Input: part model. Units: mm. Frame: model coordinates. A direction names the side the tool comes from. Coordinates: 2 decimals unless noted, no trailing zeros. Loops run counter-clockwise (first coordinate to the right, second up) from the corner with the lowest first, then second, coordinate; pieces in that order, holes last. Notation, with made-up numbers: M 31,29.5 L 36,29.5 A15 ccw 36,47.5 Z; hole C 20.5,-23.75 d4. An arc over 180 degrees is marked long. Use a Markdown table: item, result. Add a question column.
1. Section B-B on y = 0.95. Output: boundary loops of the cut face in (x, z), then the cut area to 3 significant figures.
2. Pin query (flat end, axial travel): pin 1 (18 mm diameter, centred on x = -1.5, z = 7, fed in from +Y); pin 2 (1 mm diameter, centred on y = 2.5, z = 16, fed in from +X). Return the tip coordinate at first contact, or that it passes through.
3. Line query: L1, parallel to X at y = 0.45, z = -15.25; L2, parallel to X at y = 0.35, z = -14.5. Output: solid intervals per line, ascending. Write a range as [from, to].
4. Section A-A on x = 15.25. Output: boundary loops of the cut face in (y, z).
5. Section C-C on z = -0.5. Output: boundary loops of the cut face in (x, y).
6. Set-up query: faces 5 (the flat face through (9, 3, 14.998)), 6 (the cylindrical face through (-16.75, 0.86, 15.18)). Return all of +Z, -Z, +X, -X, +Y, -Y with unobstructed straight access to the full face (end or side cutting, diameter ignored); none if empty.
7. Section D-D on x = -4.5. Output: boundary loops of the cut face in (y, z), then the cut area to 3 significant figures.
8. Draft query along X for faces 1 (the cylindrical face through (-17.43, 0.86, -17.4)), 2 (the flat face through (0, 1, 18)), 3 (the flat face through (9, 1.85, 17)), 4 (the cylindrical face through (17.4, 0.86, -17.43)). Return one class per face: +X half, -X half, draft (parallel to the pull), parting line (faces both ways), or undercut.
```python
from build123d import *

# Parameters (mm, degrees)
SKETCH1_R           = 1.5
BOSS_EXTRUDE3_DEPTH = 1.75
BOSS_EXTRUDE4_DEPTH = 3.00210529
BOSS_EXTRUDE5_DEPTH = 0.5


with BuildPart() as part:
    # Sketch1 → Boss-Extrude3 (new body)
    with BuildSketch(Plane(origin=(0, 0, 0), x_dir=(1, 0, 0), z_dir=(0, 1, 0))):
        with BuildLine():
            Line((16, -18), (-16, -18))
            ThreePointArc((-16, -18), (-17.414213562, -17.414213562), (-18, -16))
            Line((-18, -16), (-18, 16))
            ThreePointArc((-18, 16), (-17.414213562, 17.414213562), (-16, 18))
            Line((-16, 18), (16, 18))
            ThreePointArc((16, 18), (17.414213562, 17.414213562), (18, 16))
            Line((18, 16), (18, -16))
            ThreePointArc((18, -16), (17.414213562, -17.414213562), (16, -18))
        make_face()
        with Locations((-15.25, 15.25)):
            Circle(SKETCH1_R, mode=Mode.SUBTRACT)
        with Locations((15.25, 15.25)):
            Circle(SKETCH1_R, mode=Mode.SUBTRACT)
        with Locations((15.25, -15.25)):
            Circle(SKETCH1_R, mode=Mode.SUBTRACT)
        with Locations((-15.25, -15.25)):
            Circle(SKETCH1_R, mode=Mode.SUBTRACT)
    extrude(amount=BOSS_EXTRUDE3_DEPTH)

    # Sketch6 → Boss-Extrude4 (add)
    with BuildSketch(Plane(origin=(-4.326463131, 0, 18), x_dir=(1, 0, 0), z_dir=(0, 0, 1))):
        with BuildLine():
            Line((11.230523664, 1.75), (15.230523664, 1.75))
            Line((15.230523664, 1.75), (15.230523664, 3.050219677))
            ThreePointArc((15.230523664, 3.050219677), (15.17194502, 3.191641033), (15.030523664, 3.250219677))
            Line((15.030523664, 3.250219677), (14.680523664, 3.250219677))
            ThreePointArc((14.680523664, 3.250219677), (14.539102307, 3.308798321), (14.480523664, 3.450219677))
            Line((14.480523664, 3.450219677), (14.480523664, 3.55))
            ThreePointArc((14.480523664, 3.55), (14.42194502, 3.691421356), (14.280523664, 3.75))
            Line((14.280523664, 3.75), (12.180523664, 3.75))
            ThreePointArc((12.180523664, 3.75), (12.039102307, 3.691421356), (11.980523664, 3.55))
            Line((11.980523664, 3.55), (11.980523664, 3.450219677))
            ThreePointArc((11.980523664, 3.450219677), (11.92194502, 3.308798321), (11.780523664, 3.250219677))
            Line((11.780523664, 3.250219677), (11.430523664, 3.250219677))
            ThreePointArc((11.430523664, 3.250219677), (11.289102307, 3.191641033), (11.230523664, 3.050219677))
            Line((11.230523664, 3.050219677), (11.230523664, 1.75))
        make_face()
        with BuildLine():
            Line((12.180523664, 3.65), (14.280523664, 3.65))
            ThreePointArc((14.280523664, 3.65), (14.351234342, 3.620710678), (14.380523664, 3.55))
            Line((14.380523664, 3.55), (14.380523664, 3.450219677))
            ThreePointArc((14.380523664, 3.450219677), (14.468391629, 3.238087642), (14.680523664, 3.150219677))
            Line((14.680523664, 3.150219677), (15.030523664, 3.150219677))
            ThreePointArc((15.030523664, 3.150219677), (15.101234342, 3.120930355), (15.130523664, 3.050219677))
            Line((15.130523664, 3.050219677), (15.130523664, 1.85))
            Line((15.130523664, 1.85), (11.330523664, 1.85))
            Line((11.330523664, 1.85), (11.330523664, 3.050219677))
            ThreePointArc((11.330523664, 3.050219677), (11.359812985, 3.120930355), (11.430523664, 3.150219677))
            Line((11.430523664, 3.150219677), (11.780523664, 3.150219677))
            ThreePointArc((11.780523664, 3.150219677), (11.992655698, 3.238087642), (12.080523664, 3.450219677))
            Line((12.080523664, 3.450219677), (12.080523664, 3.55))
            ThreePointArc((12.080523664, 3.55), (12.109812985, 3.620710678), (12.180523664, 3.65))
        make_face(mode=Mode.SUBTRACT)
    extrude(amount=-BOSS_EXTRUDE4_DEPTH)

    # Sketch7 → Boss-Extrude5 (add)
    with BuildSketch(Plane(origin=(0, 0, 14.99789471), x_dir=(-1, 0, 0), z_dir=(0, 0, -1))):
        with BuildLine():
            Line((-6.904060533, 1.75), (-6.904060533, 3.050219677))
            ThreePointArc((-6.904060533, 3.050219677), (-6.962639176, 3.191641033), (-7.104060533, 3.250219677))
            Line((-7.104060533, 3.250219677), (-7.454060533, 3.250219677))
            ThreePointArc((-7.454060533, 3.250219677), (-7.595481889, 3.308798321), (-7.654060533, 3.450219677))
            Line((-7.654060533, 3.450219677), (-7.654060533, 3.55))
            ThreePointArc((-7.654060533, 3.55), (-7.712639176, 3.691421356), (-7.854060533, 3.75))
            Line((-7.854060533, 3.75), (-9.954060533, 3.75))
            ThreePointArc((-9.954060533, 3.75), (-10.095481889, 3.691421356), (-10.154060533, 3.55))
            Line((-10.154060533, 3.55), (-10.154060533, 3.450219677))
            ThreePointArc((-10.154060533, 3.450219677), (-10.212639176, 3.308798321), (-10.354060533, 3.250219677))
            Line((-10.354060533, 3.250219677), (-10.704060533, 3.250219677))
            ThreePointArc((-10.704060533, 3.250219677), (-10.845481889, 3.191641033), (-10.904060533, 3.050219677))
            Line((-10.904060533, 3.050219677), (-10.904060533, 1.75))
            Line((-10.904060533, 1.75), (-6.904060533, 1.75))
        make_face()
    extrude(amount=BOSS_EXTRUDE5_DEPTH)


solid = part.part
```
Answers below:
| question | item | result |
|---|---|---|
| 1 | outline | M -18,-16 A2 ccw -16,-18 L 16,-18 A2 ccw 18,-16 L 18,16 A2 ccw 16,18 L -16,18 A2 ccw -18,16 Z; hole C -15.25,-15.25 d3; hole C -15.25,15.25 d3; hole C 15.25,-15.25 d3; hole C 15.25,15.25 d3 |
| 1 | area | 1,260 mm² |
| 2 | pin 1 | stops at y = 1.75 |
| 2 | pin 2 | stops at x = 10.9 |
| 3 | L1 | x = [-18, -16.75], [-13.75, 13.75], [16.75, 18] |
| 3 | L2 | x = [-18, -16.55], [-13.95, 13.95], [16.55, 18] |
| 4 | outline | M 0,-18 L 1.75,-18 L 1.75,-16.75 L 0,-16.75 Z; M 0,-13.75 L 1.75,-13.75 L 1.75,13.75 L 0,13.75 Z; M 0,16.75 L 1.75,16.75 L 1.75,18 L 0,18 Z |
| 5 | outline | M -18,0 L 18,0 L 18,1.75 L -18,1.75 Z |
| 6 | face 5 | +Z |
| 6 | face 6 | +Y, -Y |
| 7 | outline | M 0,-18 L 1.75,-18 L 1.75,18 L 0,18 Z |
| 7 | area | 63.0 mm² |
| 8 | face 1 | -X half |
| 8 | face 2 | draft |
| 8 | face 3 | undercut |
| 8 | face 4 | +X half |
